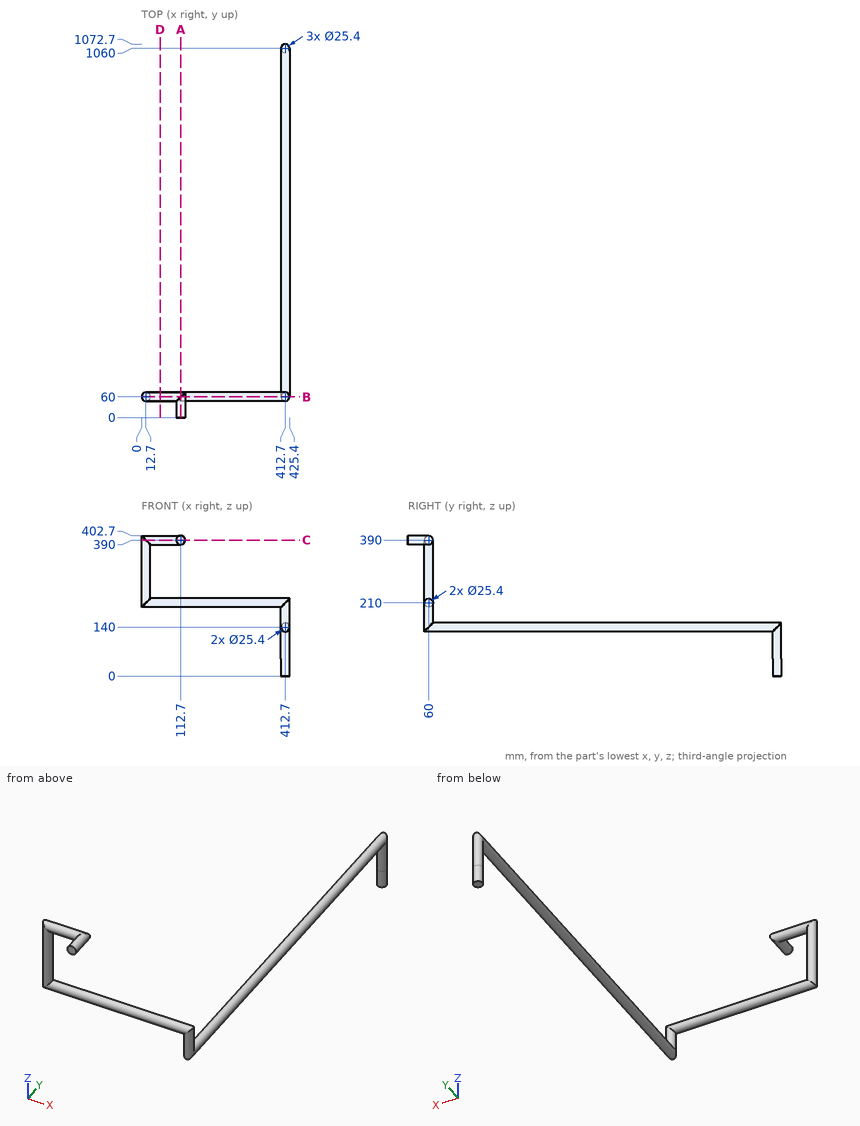
For this review, use the dimensioned drawing (mm, ordinates from the lowest corner) and the shaded views. Coordinates: 2 decimals unless noted, no trailing zeros. Order: outer loops, then holes, each group sorted by start corner. A loop starts at its lowest first (then second) coordinate and runs counter-clockwise, first axis right, second up. Notation, with made-up numbers: (86, -13) - (131, -13) arc R25 cw to (131, 12) - close; hole circle Ø11 at (74.5, 9.25). An arc over 180 degrees is marked (long way). Answer as a JSON object with one key per item and string values. Group by question number.
1. We need section C-C on z = 390. State the section outline as (x, y) points, then the cut area to 3 significant figures.
2. We need section B-B on y = 60. State the section outline as (x, z) points, then the cut area to 3 significant figures.
3. For probe 1 along Y at (x, z) = (274, 208.5); probe 2 along X at (y, z) = (368, 137), list the stretches that pass through material, from the lowest coordinate up.
4. We need section D-D on x = 53. State the section outline as (y, z) points, then the cut area to 3 significant figures.
5. We need section A-A on x = 112.7. State the section outline as (y, z) points, then the cut area to 3 significant figures.
6. Clearance check with a flat-ended pin moving along its axis: P1, Ø12, axis at y = 688.5, z = 151.5, coming from the -X side. State where the tip first meets the part, or that it passes through.
Final values:
{
 "1": {"outline": "(12.7, 47.3) - (100, 47.3) - (100, 0) - (125.4, 0) - (125.4, 72.7) - (12.7, 72.7) arc R12.7 ccw to start", "area": "4,320 mm²"},
 "2": {"outline": "(0, 197.3) - (400, 197.3) - (400, 140) arc R12.7 ccw to (425.4, 140) - (425.4, 222.7) - (25.4, 222.7) - (25.4, 377.3) - (112.7, 377.3) arc R12.7 ccw to (112.7, 402.7) - (0, 402.7) - close", "area": "19,600 mm²"},
 "3": {"probe 1": "47.39 to 72.61", "probe 2": "400.36 to 425.04"},
 "4": {"outline": "circle Ø25.4 at (60, 210); circle Ø25.4 at (60, 390)", "area": "1,010 mm²"},
 "5": {"outline": "(0, 377.3) - (60, 377.3) arc R12.7 ccw to (60, 402.7) - (0, 402.7) - close; circle Ø25.4 at (60, 210)", "area": "2,280 mm²"},
 "6": {"P1": "x = 401.25"}
}
